Geometry check sheet. Reference: the model listing, model coordinates, mm. Coordinates: 2 decimals unless noted, no trailing zeros. Write each loop counter-clockwise with the first axis right and the second up, starting at its lowest first coordinate (ties: lowest second). Pieces come first, ordered by that corner, then holes. Notation, with made-up numbers: (-6, 68) -> (37, 68) arc R26 ccw to (37, 100) -> close; hole circle Ø8 at (46, 33). An arc over 180 degrees is marked (long way). Answer in a Markdown table with one row per item. Add a question column.
1. Scan lines: L1, parallel to Z at x = 47.5, y = 0.4; L2, parallel to X at y = 0.55, z = -2.5; L3, parallel to Y at x = 47.5, z = -4.25. Record each from-to range of solid material in increasing order. Write a range as from..to.
2. Cross-section at B-B on z = -2.5. Record the cut outline in (x, y).
3. Depth check by flat-ended pin: P1, Ø3, axis at x = 47.5, z = -2.5, coming from the -Y side; P2, Ø3, axis at x = 47.5, z = -22.5, coming from the +Y side. Enter the tip coordinate at first touch or a pass-through.
4. Cross-section at A-A on x = 2.5. Record the cut outline in (y, z).
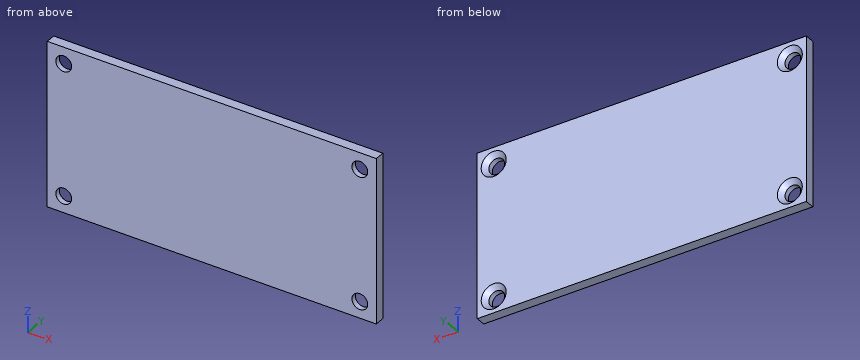
```python
from build123d import *

# Parameters (mm, degrees)
SKETCH_1_W                  = 50
SKETCH_1_H                  = 25
EXTRUDE_1_DEPTH             = 1.5
PATTERN_LINEAR_1_COUNT      = 2
PATTERN_LINEAR_1_PITCH      = 45
PATTERN_LINEAR_1_COUNT_DIR2 = 2
PATTERN_LINEAR_1_PITCH_DIR2 = 20


with BuildPart() as part:
    # 草图1 → 凸台-拉伸1 (new body)
    with BuildSketch(Plane(origin=(0, 0, 0), x_dir=(1, 0, 0), z_dir=(0, 1, 0))):
        with Locations((25, 12.5)):
            Rectangle(SKETCH_1_W, SKETCH_1_H)
    extrude(amount=EXTRUDE_1_DEPTH)

    # 草图3 → M2 平头机械螺钉的锥形沉头孔1 (revolve, cut)
    with BuildSketch(Plane(origin=(2.5, 1.5, -22.5), x_dir=(0, 0, 1), z_dir=(1, 0, 0))):
        Polygon((0, 0), (0, 8.721032743), (1.2, 8), (1.2, 0.7), (1.9, 0), align=None)
    hole_wizard_m2_1 = revolve(axis=Axis((2.5, 7.85, -22.5), (0, -1, 0)), mode=Mode.SUBTRACT)

    # 阵列(线性)1: Hole Wizard M2 _1 2 × 2
    with Locations(*[(i * PATTERN_LINEAR_1_PITCH, 0, j * PATTERN_LINEAR_1_PITCH_DIR2) for i in range(PATTERN_LINEAR_1_COUNT) for j in range(PATTERN_LINEAR_1_COUNT_DIR2) if (i, j) != (0, 0)]):
        add(hole_wizard_m2_1, mode=Mode.SUBTRACT)


solid = part.part
```
Results found:
| question | item | result |
|---|---|---|
| 1 | L1 | z = -25..-23.7, -21.3..-3.7, -1.3..0 |
| 1 | L2 | x = 0..1.3, 3.7..46.3, 48.7..50 |
| 1 | L3 | y = 0..1.35 |
| 2 | outline | (0, 0) -> (1.3, 0) -> (1.3, 0.8) -> (0.6, 1.5) -> (0, 1.5) -> close; (3.7, 0) -> (46.3, 0) -> (46.3, 0.8) -> (45.6, 1.5) -> (4.4, 1.5) -> (3.7, 0.8) -> close; (48.7, 0) -> (50, 0) -> (50, 1.5) -> (49.4, 1.5) -> (48.7, 0.8) -> close |
| 3 | P1 | stops at y = 0 |
| 3 | P2 | stops at y = 1.1 |
| 4 | outline | (0, -25) -> (1.5, -25) -> (1.5, -24.4) -> (0.8, -23.7) -> (0, -23.7) -> close; (0, -21.3) -> (0.8, -21.3) -> (1.5, -20.6) -> (1.5, -4.4) -> (0.8, -3.7) -> (0, -3.7) -> close; (0, -1.3) -> (0.8, -1.3) -> (1.5, -0.6) -> (1.5, 0) -> (0, 0) -> close |
